For this review, take the finished solid that the model builds, in its own axes (mm). A direction names the side the tool comes from. Coordinates: 2 decimals unless noted, no trailing zeros. Order: outer loops, then holes, each group sorted by start corner. A loop starts at its lowest first (then second) coordinate and runs counter-clockwise, first axis right, second up. Notation, with made-up numbers: (51, 81) -> (59, 81) arc R23 cw to (59, 95) -> close; hole circle Ø10 at (49.5, 24.5). An arc over 180 degrees is marked (long way). Answer as a JSON object with one key per item and string values. Group by question number.
1) Add section A-A, the plane z = -15.25. Write out the cut boundary in (x, y), then the cut area to 3 significant figures.
2) Add section D-D, the plane z = 13. Write out the cut boundary in (x, y).
3) Draft analysis for pull direction X (two halves, no side actions). For faces 4 (the cylindrical face through (-17.43, 0.86, -17.4)), 5 (the cylindrical face through (13.75, 0.86, -15.32)), 6 (the flat face through (0, 1.75, 0)), state which applies: +X half, -X half, draft (parallel to the pull), parting line (faces both ways), or undercut.
4) Add section B-B, the plane y = 0.6. Write out the cut boundary in (x, z).
5) Machinability: for faces 1 (the flat face through (8, 2, 14.5)), 2 (the flat face through (8, 3, 15)), 3 (the cylindrical face through (-17.4, 0.86, 17.43)), which of the approach directions +Z, -Z, +X, -X, +Y, -Y give a long, thin tool a straight path to every point of the face, cutting with its end or side? Answer none if there is none.
6) Wall thickness on L1, parallel to Z at x = -15.25, y = 0.6; L2, parallel to X at y = 1.7, z = -14: over which ranges is each line inside the solid? List them lowest first.
7) Add section C-C, the plane x = -15. Write out the cut boundary in (y, z), then the cut area to 3 significant figures.
8) For pin 1 (1 mm diameter, centred on y = 2, z = 17, fed in from -X); pin 2 (8 mm diameter, centred on x = 11, z = 8, fed in from +Y), all flat-tipped, find the tip position at first contact; note any pin that passes through.
from build123d import *

# Parameters (mm, degrees)
SKETCH1_R           = 1.5
BOSS_EXTRUDE2_DEPTH = 1.75
BOSS_EXTRUDE3_DEPTH = 3
BOSS_EXTRUDE4_DEPTH = 0.5
SKETCH5_R           = 0.210276494
CUT_EXTRUDE1_DEPTH  = 0.5


with BuildPart() as part:
    # Sketch1 → Boss-Extrude2 (new body)
    with BuildSketch(Plane(origin=(0, 0, 0), x_dir=(1, 0, 0), z_dir=(0, 1, 0))):
        with BuildLine():
            Line((-16, 18), (16, 18))
            ThreePointArc((16, 18), (17.414213562, 17.414213562), (18, 16))
            Line((18, 16), (18, -16))
            ThreePointArc((18, -16), (17.414213562, -17.414213562), (16, -18))
            Line((16, -18), (-16, -18))
            ThreePointArc((-16, -18), (-17.414213562, -17.414213562), (-18, -16))
            Line((-18, -16), (-18, 16))
            ThreePointArc((-18, 16), (-17.414213562, 17.414213562), (-16, 18))
        make_face()
        with Locations((-15.25, 15.25)):
            Circle(SKETCH1_R, mode=Mode.SUBTRACT)
        with Locations((15.25, 15.25)):
            Circle(SKETCH1_R, mode=Mode.SUBTRACT)
        with Locations((15.25, -15.25)):
            Circle(SKETCH1_R, mode=Mode.SUBTRACT)
        with Locations((-15.25, -15.25)):
            Circle(SKETCH1_R, mode=Mode.SUBTRACT)
    extrude(amount=BOSS_EXTRUDE2_DEPTH)

    # Sketch3 → Boss-Extrude3 (add)
    with BuildSketch(Plane.XY.offset(18)):
        with BuildLine():
            Line((6, 1.75), (10, 1.75))
            Line((10, 1.75), (10, 2.643928524))
            ThreePointArc((10, 2.643928524), (9.941421356, 2.78534988), (9.8, 2.843928524))
            Line((9.8, 2.843928524), (9.148500836, 2.843928524))
            ThreePointArc((9.148500836, 2.843928524), (9.007079479, 2.902507168), (8.948500836, 3.043928524))
            Line((8.948500836, 3.043928524), (8.948500836, 3.55))
            ThreePointArc((8.948500836, 3.55), (8.889922192, 3.691421356), (8.748500836, 3.75))
            Line((8.748500836, 3.75), (7.202410951, 3.75))
            ThreePointArc((7.202410951, 3.75), (7.060989594, 3.691421356), (7.002410951, 3.55))
            Line((7.002410951, 3.55), (7.002410951, 3.043928524))
            ThreePointArc((7.002410951, 3.043928524), (6.943832307, 2.902507168), (6.802410951, 2.843928524))
            Line((6.802410951, 2.843928524), (6.2, 2.843928524))
            ThreePointArc((6.2, 2.843928524), (6.058578644, 2.78534988), (6, 2.643928524))
            Line((6, 2.643928524), (6, 1.75))
        make_face()
        with BuildLine():
            Line((6.1, 1.85), (6.1, 2.643928524))
            ThreePointArc((6.1, 2.643928524), (6.129289322, 2.714639202), (6.2, 2.743928524))
            Line((6.2, 2.743928524), (6.802410951, 2.743928524))
            ThreePointArc((6.802410951, 2.743928524), (7.014542985, 2.83179649), (7.102410951, 3.043928524))
            Line((7.102410951, 3.043928524), (7.102410951, 3.55))
            ThreePointArc((7.102410951, 3.55), (7.131700273, 3.620710678), (7.202410951, 3.65))
            Line((7.202410951, 3.65), (8.748500836, 3.65))
            ThreePointArc((8.748500836, 3.65), (8.819211514, 3.620710678), (8.848500836, 3.55))
            Line((8.848500836, 3.55), (8.848500836, 3.043928524))
            ThreePointArc((8.848500836, 3.043928524), (8.936368801, 2.83179649), (9.148500836, 2.743928524))
            Line((9.148500836, 2.743928524), (9.8, 2.743928524))
            ThreePointArc((9.8, 2.743928524), (9.870710678, 2.714639202), (9.9, 2.643928524))
            Line((9.9, 2.643928524), (9.9, 1.85))
            Line((9.9, 1.85), (6.1, 1.85))
        make_face(mode=Mode.SUBTRACT)
    extrude(amount=-BOSS_EXTRUDE3_DEPTH)

    # Sketch4 → Boss-Extrude4 (add)
    with BuildSketch(Plane(origin=(0, 0, 15), x_dir=(-1, 0, 0), z_dir=(0, 0, -1))):
        with BuildLine():
            Line((-6, 1.75), (-10, 1.75))
            Line((-10, 1.75), (-10, 2.643928524))
            ThreePointArc((-10, 2.643928524), (-9.941421356, 2.78534988), (-9.8, 2.843928524))
            Line((-9.8, 2.843928524), (-9.148500836, 2.843928524))
            ThreePointArc((-9.148500836, 2.843928524), (-9.007079479, 2.902507168), (-8.948500836, 3.043928524))
            Line((-8.948500836, 3.043928524), (-8.948500836, 3.55))
            ThreePointArc((-8.948500836, 3.55), (-8.889922192, 3.691421356), (-8.748500836, 3.75))
            Line((-8.748500836, 3.75), (-7.202410951, 3.75))
            ThreePointArc((-7.202410951, 3.75), (-7.060989594, 3.691421356), (-7.002410951, 3.55))
            Line((-7.002410951, 3.55), (-7.002410951, 3.043928524))
            ThreePointArc((-7.002410951, 3.043928524), (-6.943832307, 2.902507168), (-6.802410951, 2.843928524))
            Line((-6.802410951, 2.843928524), (-6.2, 2.843928524))
            ThreePointArc((-6.2, 2.843928524), (-6.058578644, 2.78534988), (-6, 2.643928524))
            Line((-6, 2.643928524), (-6, 1.75))
        make_face()
    extrude(amount=BOSS_EXTRUDE4_DEPTH)

    # Sketch5 → Cut-Extrude1 (cut)
    with BuildSketch(Plane(origin=(0, 0, 14.5), x_dir=(-1, 0, 0), z_dir=(0, 0, -1))):
        with Locations((-8.596830264, 2.577355932)):
            Circle(SKETCH5_R)
        with Locations((-7.929200441, 2.577355932)):
            Circle(SKETCH5_R)
        with Locations((-7.321447194, 2.577355932)):
            Circle(SKETCH5_R)
    extrude(amount=-CUT_EXTRUDE1_DEPTH, mode=Mode.SUBTRACT)


solid = part.part
Output values:
{
 "1": {"outline": "(-18, 0) -> (-16.75, 0) -> (-16.75, 1.75) -> (-18, 1.75) -> close; (-13.75, 0) -> (13.75, 0) -> (13.75, 1.75) -> (-13.75, 1.75) -> close; (16.75, 0) -> (18, 0) -> (18, 1.75) -> (16.75, 1.75) -> close", "area": "52.5 mm²"},
 "2": {"outline": "(-18, 0) -> (18, 0) -> (18, 1.75) -> (-18, 1.75) -> close"},
 "3": {"face 4": "-X half", "face 5": "undercut", "face 6": "draft"},
 "4": {"outline": "(-18, -16) arc R2 ccw to (-16, -18) -> (16, -18) arc R2 ccw to (18, -16) -> (18, 16) arc R2 ccw to (16, 18) -> (-16, 18) arc R2 ccw to (-18, 16) -> close; hole circle Ø3 at (-15.25, -15.25); hole circle Ø3 at (-15.25, 15.25); hole circle Ø3 at (15.25, -15.25); hole circle Ø3 at (15.25, 15.25)"},
 "5": {"face 1": "-Z, +X, -X, +Y", "face 2": "+Z", "face 3": "+Z, -X, +Y, -Y"},
 "6": {"L1": "z = -18 to -16.75, -13.75 to 13.75, 16.75 to 18", "L2": "x = -18 to -16.08, -14.42 to 14.42, 16.08 to 18"},
 "7": {"outline": "(0, -18) -> (1.75, -18) -> (1.75, -16.73) -> (0, -16.73) -> close; (0, -13.77) -> (1.75, -13.77) -> (1.75, 13.77) -> (0, 13.77) -> close; (0, 16.73) -> (1.75, 16.73) -> (1.75, 18) -> (0, 18) -> close", "area": "52.6 mm²"},
 "8": {"pin 1": "stops at x = -17.92", "pin 2": "stops at y = 1.75"}
}
